The model under review builds one solid part; all positions refer to its coordinate system, in mm. A direction names the side the tool comes from. Round coordinates to 2 decimals unless told otherwise and drop trailing zeros. Write each loop counter-clockwise with the first axis right and the second up, starting at its lowest first coordinate (ties: lowest second). Pieces come first, ordered by that corner, then holes. Notation, with made-up numbers: M 43.5,84.25 L 89.5,84.25 A28 cw 89.5,106.25 Z; hole C 39,0.5 d4. An arc over 180 degrees is marked long. One line per item, written item: value. Start each with the question number.
1) For P1, Ø17, axis at y = 0, z = 3.5, coming from the -X side; P2, Ø8, axis at x = 288, z = 16.5, coming from the +Y side; P3, Ø1, axis at x = 120, y = -15.5, coming from the -Z side; P4, Ø10, axis at x = 138.5, z = -4, coming from the -Y side, all flat-tipped, find the tip position at first contact; note any pin that passes through.
2) Take a section at B-B, the plane x = 247.5. Write out the cut boundary in (y, z), and give its area (3 significant figures).
3) Tool access review of faces 4 (the face through (35.5, -10, -3.2)), 5 (the face through (72, -11, 0)), 6 (the face through (90.202, 116.812, 0.042)), 7 (the face through (73.09, 82.07, 1.17)), 8 (the face through (455, 0, 0)): name each direction out of +Z, -Z, +X, -X, +Y, -Y from which nothing blocks a thin tool from reaching the whole face with its end or side.
4) Take a section at A-A, the plane y = 73. Write out the cut boundary in (x, z).
5) Wall thickness on probe 1 along Z at (x, y) = (19, 0); probe 2 along X at (y, z) = (11.5, -5.5); probe 3 along X at (y, z) = (89.5, 0): over which ranges is each line inside the solid? List them lowest first.
6) Mouldability with a two-part tool opening along Y and no side actions: class faces 1 (the face through (452.524, 4.708, 21.201)), 2 (the face through (213, -37.1, 15.4)), 3 (the face through (331.64, 39.96, -1.76)) as +Y half, -Y half, draft (parallel to the pull), parting line (faces both ways), or undercut.
from build123d import *

# Parameters (mm, degrees)
SKETCH2_W          = 1
SKETCH2_H          = 88
CUT_EXTRUDE1_DEPTH = 10


with BuildPart() as part:
    # Sketch1 → Revolve1 (revolve)
    with BuildSketch(Plane.XY, mode=Mode.PRIVATE) as revolve1_sk:
        with BuildLine():
            Line((0, 12.5), (70, 12.5))
            Line((70, 12.5), (70, 16.864606255))
            ThreePointArc((70, 16.864606255), (70.010085496, 17.499679587), (70.040331814, 18.134112416))
            Line((70.040331814, 18.134112416), (71.014116135, 33.444327156))
            ThreePointArc((71.014116135, 33.444327156), (73.209921196, 38.104424066), (78, 40))
            Line((78, 40), (193, 40))
            Line((193, 40), (193, 42))
            Line((193, 42), (213, 42))
            Line((213, 42), (213, 40))
            Line((213, 40), (447, 40))
            ThreePointArc((447, 40), (450.195681655, 38.845467301), (451.915555723, 35.915047504))
            Line((451.915555723, 35.915047504), (454.662222892, 21.160190017))
            ThreePointArc((454.662222892, 21.160190017), (454.915376695, 19.337871346), (455, 17.5))
            Line((455, 17.5), (455, 0))
            Line((455, 0), (453, 0))
            Line((453, 0), (453, 17.5))
            ThreePointArc((453, 17.5), (452.923839026, 19.154084211), (452.696000602, 20.794171015))
            Line((452.696000602, 20.794171015), (449.949333434, 35.549028503))
            ThreePointArc((449.949333434, 35.549028503), (448.917408993, 37.30728038), (447, 38))
            Line((447, 38), (78, 38))
            ThreePointArc((78, 38), (74.57851514, 36.64601719), (73.010082953, 33.31737654))
            Line((73.010082953, 33.31737654), (72.036298632, 18.0071618))
            ThreePointArc((72.036298632, 18.0071618), (72.009076947, 17.436172254), (72, 16.864606255))
            Line((72, 16.864606255), (72, 10.5))
            Line((72, 10.5), (0, 10.5))
            Line((0, 10.5), (0, 12.5))
        make_face()
    revolve(revolve1_sk.sketch.rotate(Axis((0, 0, 0), (1, 0, 0)), 180), axis=Axis((0, 0, 0), (1, 0, 0)))

    # Sketch2 → Revolve2 (revolve)
    with BuildSketch(Plane.XY, mode=Mode.PRIVATE) as revolve2_sk:
        with Locations((73.514116135, 81)):
            Rectangle(SKETCH2_W, SKETCH2_H)
    revolve(revolve2_sk.sketch.rotate(Axis((82.014116135, 37, 0), (0, 1, 0)), 270), axis=Axis((82.014116135, 37, 0), (0, 1, 0)))

    # Sketch3 → Cut-Extrude1 (cut, symmetric)
    with BuildSketch(Plane.XY):
        Polygon((82.014116135, 125), (91.014116135, 125), (91.014116135, 116), align=None)
    extrude(amount=CUT_EXTRUDE1_DEPTH, both=True, mode=Mode.SUBTRACT)

    # Sketch4 → Revolve3 (revolve)
    with BuildSketch(Plane(origin=(0, 0, 0), x_dir=(1, 0, 0), z_dir=(0, 1, 0))):
        Polygon((74.509274782, -28.686334103), (55.456715899, -39.686334103), (55.956715899, -40.552359507), (75.009274782, -29.552359507), align=None)
    revolve(axis=Axis((53.206715899, 0, 35.789219786), (0.8660254037844379, 0, -0.5000000000000013)))


solid = part.part
Checked values:
1. P1: stops at x = 0
1. P2: stops at y = 38
1. P3: stops at z = -37.08
1. P4: stops at y = -40
2. outline: C 0,0 d80; hole C 0,0 d76
2. area: 490 mm2
3. face 4: -X
3. face 5: none
3. face 6: +Z, -Z, +X, +Y
3. face 7: +Y
3. face 8: +Z, -Z, +X, +Y, -Y
4. outline: C 82.01,0 d18; hole C 82.01,0 d16
5. probe 1: z = -12.5 to -10.5, 10.5 to 12.5
5. probe 2: x = 70 to 72, 453 to 455
5. probe 3: x = 73.01 to 74.01, 90.01 to 91.01
6. face 1: undercut
6. face 2: draft
6. face 3: parting line
